Can you work these out from the model? Positions are in its coordinate system, mm. Coordinates: 2 decimals unless noted, no trailing zeros. Loops run counter-clockwise (first coordinate to the right, second up) from the corner with the lowest first, then second, coordinate; pieces in that order, holes last.
```python
from build123d import *

# Parameters (mm, degrees)
BOSS_EXTRUDE1_DEPTH = 9.525
SKETCH2_R           = 4.7625
SKETCH2_R_2         = 2.3749
CUT_EXTRUDE1_DEPTH  = 9.525
FILLET1_R           = 2.54


with BuildPart() as part:
    # Sketch1 → Boss-Extrude1 (new body)
    with BuildSketch(Plane.XY):
        with BuildLine():
            ThreePointArc((4.57280399, 15.202140924), (0, 15.875), (-4.57280399, 15.202140924))
            ThreePointArc((-4.57280399, 15.202140924), (-8.467578202, 6.295312552), (-15.875, 0))
            ThreePointArc((-15.875, 0), (0, -15.875), (15.875, 0))
            ThreePointArc((15.875, 0), (8.467578202, 6.295312552), (4.57280399, 15.202140924))
        make_face()
    extrude(amount=BOSS_EXTRUDE1_DEPTH)

    # Sketch2 → Cut-Extrude1 (cut)
    with BuildSketch(Plane.XY.offset(9.525)):
        Circle(SKETCH2_R)
        with Locations((0, 9.525)):
            Circle(SKETCH2_R_2)
    extrude(amount=-CUT_EXTRUDE1_DEPTH, mode=Mode.SUBTRACT)

    # Fillet1
    fillet1_edges = [part.edges().sort_by_distance(p)[0] for p in [
        (-8.467578202, 6.295312552, 9.525),
        (0, -15.875, 9.525),
        (8.467578202, 6.295312552, 9.525),
        (0, -15.875, 0),
        (-8.467578202, 6.295312552, 0),
        (0, 15.875, 0),
        (8.467578202, 6.295312552, 0),
        (0, 15.875, 9.525),
    ]]
    fillet(fillet1_edges, radius=FILLET1_R)


solid = part.part
```
(1) If I drill on probe 1 along Y at (x, z) = (1, 2.75); probe 2 along X at (y, z) = (8, 4); probe 3 along X at (y, z) = (11.5, 4.25), over which ranges is the centre line in solid material (lowest first)?
Check values:
probe 1: y = -15.84 to -4.66, 4.66 to 7.37, 11.68 to 15.84
probe 2: x = -7.32 to -1.82, 1.82 to 7.32
probe 3: x = -5.61 to -1.32, 1.32 to 5.61
(2) If we mould it in two halves opening along Y, with no side actions, what happens to faces 1 (the cylindrical face through (-8.386, 6.406, 4.731)), 2 (the cylindrical face through (-0.515, 7.207, 4.829)), 3 (the cylindrical face through (-3.78, -2.9, 4.83)), 4 (the cylindrical face through (-0.35, -15.87, 4.73))? For each: released by +Y, released by -Y, zero draft, split by the parting line, or undercut.
Check values:
face 1: released by +Y
face 2: undercut
face 3: undercut
face 4: released by -Y
(3) I want a section at B-B on z = 6.5. State how many separate pieces and enclosed holes the cut face has, then the cut area to 3 significant figures.
Check values:
separate pieces: 1
enclosed holes: 2
area: 566 mm2
(4) I want a section at A-A on x = 0. Write out the boundary of the cut face in (y, z) (1 decimal).
Check values:
outline: (-15.9, 2.5) arc R2.5 ccw to (-13.3, 0) - (-4.8, 0) - (-4.8, 9.5) - (-13.3, 9.5) arc R2.5 ccw to (-15.9, 7) - close; (4.8, 0) - (7.2, 0) - (7.2, 9.5) - (4.8, 9.5) - close; (11.9, 0) - (13.3, 0) arc R2.5 ccw to (15.9, 2.5) - (15.9, 7) arc R2.5 ccw to (13.3, 9.5) - (11.9, 9.5) - close
(5) I'm going to push flat-ended pins straight in: pin 1 (2 mm diameter, centred on x = -4.5, z = 8, fed in from +Y); pin 2 (5.5 mm diameter, centred on x = 0, y = 0, fed in from -Z); pin 3 (3 mm diameter, centred on y = -12, z = 3, fed in from -X). Where does each tip first touch, or does it pass through?
Check values:
pin 1: stops at y = 15.4
pin 2: passes through
pin 3: stops at x = -11.91
